Design review of the part built by this model. Coordinates are the model's own, in mm. A direction names the side the tool comes from. Give positions to 0.01 mm unless a question says otherwise; leave off trailing zeros. Write each loop counter-clockwise with the first axis right and the second up, starting at its lowest first coordinate (ties: lowest second). Pieces come first, ordered by that corner, then holes. Notation, with made-up numbers: (1, 76) -> (30, 76) arc R27 ccw to (30, 100) -> close; hole circle Ø9 at (28, -39.5). An arc over 180 degrees is marked (long way). Return JSON: item names as keys, results as strings. Group by question number.
from build123d import *

# Parameters (mm, degrees)
SKETCH1_W           = 100
SKETCH1_H           = 100
BOSS_EXTRUDE1_DEPTH = 25
SKETCH4_W           = 80
SKETCH4_H           = 80
CUT_EXTRUDE2_DEPTH  = 40
SKETCH5_R           = 7.5
CUT_EXTRUDE3_DEPTH  = 100
BOSS_EXTRUDE4_DEPTH = 10
BOSS_EXTRUDE5_DEPTH = 10


with BuildPart() as part:
    # Sketch1 → Boss-Extrude1 (new body, symmetric)
    with BuildSketch(Plane(origin=(0, 0, 0), x_dir=(1, 0, 0), z_dir=(0, 1, 0))):
        Rectangle(SKETCH1_W, SKETCH1_H)
    extrude(amount=BOSS_EXTRUDE1_DEPTH, both=True)

    # Sketch4 → Cut-Extrude2 (cut)
    with BuildSketch(Plane(origin=(0, 25, 0), x_dir=(1, 0, 0), z_dir=(0, 1, 0))):
        Rectangle(SKETCH4_W, SKETCH4_H)
    extrude(amount=-CUT_EXTRUDE2_DEPTH, mode=Mode.SUBTRACT)

    # Sketch5 → Cut-Extrude3 (cut)
    with BuildSketch(Plane.XY.offset(50)):
        with Locations((0, 25)):
            Circle(SKETCH5_R)
    extrude(amount=-CUT_EXTRUDE3_DEPTH, mode=Mode.SUBTRACT)

    # Sketch7 → Boss-Extrude4 (add)
    with BuildSketch(Plane.ZY.offset(50)):
        Polygon((-45, 33.660254038), (-50, 25), (-40, 25), align=None)
        Polygon((-35, 33.660254038), (-40, 25), (-30, 25), align=None)
        Polygon((-25, 33.660254038), (-30, 25), (-20, 25), align=None)
        Polygon((-15, 33.660254038), (-20, 25), (-10, 25), align=None)
        Polygon((-5, 33.660254038), (-10, 25), (0, 25), align=None)
        Polygon((5, 33.660254038), (0, 25), (10, 25), align=None)
        Polygon((15, 33.660254038), (10, 25), (20, 25), align=None)
        Polygon((25, 33.660254038), (20, 25), (30, 25), align=None)
        Polygon((35, 33.660254038), (30, 25), (40, 25), align=None)
        Polygon((45, 33.660254038), (40, 25), (50, 25), align=None)
    extrude(amount=-BOSS_EXTRUDE4_DEPTH)

    # Sketch8 → Boss-Extrude5 (add)
    with BuildSketch(Plane(origin=(50, 0, 0), x_dir=(0, 0, -1), z_dir=(1, 0, 0))):
        Polygon((-45, 33.660254038), (-50, 25), (-40, 25), align=None)
        Polygon((-35, 33.660254038), (-40, 25), (-30, 25), align=None)
        Polygon((-25, 33.660254038), (-30, 25), (-20, 25), align=None)
        Polygon((-15, 33.660254038), (-20, 25), (-10, 25), align=None)
        Polygon((-5, 33.660254038), (-10, 25), (0, 25), align=None)
        Polygon((5, 33.660254038), (0, 25), (10, 25), align=None)
        Polygon((15, 33.660254038), (10, 25), (20, 25), align=None)
        Polygon((25, 33.660254038), (20, 25), (30, 25), align=None)
        Polygon((35, 33.660254038), (30, 25), (40, 25), align=None)
        Polygon((50, 25), (40, 25), (45, 33.660254038), align=None)
    extrude(amount=-BOSS_EXTRUDE5_DEPTH)


solid = part.part
Q1. Mouldability with a two-part tool opening along Z and no side actions: class faces 1 (the face through (-1, -25, -1)), 2 (the face through (45.07, 29.391, 47.465)), 3 (the face through (-45.07, 29.391, 42.535)) as +Z half, -Z half, draft (parallel to the pull), parting line (faces both ways), or undercut.
Q2. Take a section at B-B, the plane y = -5.5. Give the boundary of the cut face in (x, z).
Q3. Insertion check: pin 1 (8 mm diameter, centred on x = -25.5, z = 46.5, fed in from +Y); pin 2 (2.5 mm diameter, centred on y = 31.5, z = 43, fed in from +X); pin 3 (5 mm diameter, centred on x = 28, z = -27.5, fed in from +Y). Each pin has a flat end and moves straight along its axis. Give the tip position at first contact, or say it passes through.
Q4. Take a section at A-A, the plane x = 0. Give the boundary of the cut face in (y, z), plus the area to 3 significant figures.
Q5. Take a section at C-C, the plane z = -1.5. Give the boundary of the cut face in (x, y), plus the area to 3 significant figures.
Q6. Tool access review of faces 4 (the face through (-50, 5, -1)), 5 (the face through (24, 25, -45)), 6 (the face through (40, 10, 1)), 7 (the face through (-45.07, 29.391, -17.465)): name each direction out of +Z, -Z, +X, -X, +Y, -Y from which nothing blocks a thin tool from reaching the whole face with its end or side.
Q7. For L1, parallel to X at y = -3.5, z = -27; L2, parallel to Y at x = 32, z = 37.5, list the stretches that pass through material, from the lowest coordinate up. Write a range as from..to.
Final values:
{
 "1": {"face 1": "draft", "face 2": "+Z half", "face 3": "undercut"},
 "2": {"outline": "(-50, -50) -> (50, -50) -> (50, 50) -> (-50, 50) -> close; hole (-40, -40) -> (40, -40) -> (40, 40) -> (-40, 40) -> close"},
 "3": {"pin 1": "stops at y = 25", "pin 2": "stops at x = 50", "pin 3": "stops at y = -15"},
 "4": {"outline": "(-25, -50) -> (17.5, -50) -> (17.5, -40) -> (-15, -40) -> (-15, 40) -> (17.5, 40) -> (17.5, 50) -> (-25, 50) -> close", "area": "1,650 mm²"},
 "5": {"outline": "(-50, -25) -> (50, -25) -> (50, 27.6) -> (40, 27.6) -> (40, -15) -> (-40, -15) -> (-40, 27.6) -> (-50, 27.6) -> close", "area": "1,850 mm²"},
 "6": {"face 4": "+Z, -Z, -X, +Y, -Y", "face 5": "+Z, -Z, +Y", "face 6": "+Y", "face 7": "+X, -X, +Y"},
 "7": {"L1": "x = -50..-40, 40..50", "L2": "y = -25..-15"}
}
